Autodesk Inventor part; units mm, degrees
ref_plane "YZ Plane" through (0, 0, 0) normal (1, 0, 0) x (0, 1, 0)
ref_plane "XZ Plane" through (0, 0, 0) normal (0, 1, 0) x (-1, 0, 0)
ref_plane "XY Plane" through (0, 0, 0) normal (0, 0, 1) x (1, 0, 0)
sketch "Sketch1" plane through (0, 0, 0) normal (0, 1, 0) x (-1, 0, 0)
  line L0 (-20, 20) -> (20, 20)
  line L1 (20, 20) -> (20, -20)
  line L2 (20, -20) -> (-20, -20)
  line L3 (-20, -20) -> (-20, 20)
  line L4 (-20, 20) -> (20, -20) construction
  line L5 (20, 20) -> (-20, -20) construction
  line L6 (18, 18) -> (-18, 18)
  line L7 (-18, 18) -> (-18, -18)
  line L8 (-18, -18) -> (18, -18)
  line L9 (18, -18) -> (18, 18)
  point P0 (0, 0)
  dimension "d19" = 40
  dimension "d20" = 40
  dimension "d21" = 2
extrude "Extrusion1" add sketch "Sketch1" along normal blind 460
equation "\"BendRadius\" = Thickness"
equation "\"BendReliefWidth\" = Thickness"
equation "\"BendReliefDepth\" = 0.5 * Thickness"
equation "\"TransitionRadius\" = BendRadius"
equation "\"JacobiRadiusSize\" = BendRadius"
equation "\"GapSize\" = Thickness"
properties part number "ДМФ 033 держатель лотка v2.0"
Geometry check sheet. Reference: the model listing, model coordinates, mm. A direction names the side the tool comes from. Coordinates: 2 decimals unless noted, no trailing zeros. Order: outer loops, then holes, each group sorted by start corner. A loop starts at its lowest first (then second) coordinate and runs counter-clockwise, first axis right, second up. Notation, with made-up numbers: (21.5, 23) - (51.5, 23) arc R35 ccw to (51.5, 56) - close; hole circle Ø4 at (-5, 55). An arc over 180 degrees is marked (long way). Use one line per item in the form item = value.
1. Scan line: line 1 (Z direction, x = -4, y = 357). Record every from-to range of solid material in increasing order.
Here are the results:
line_1 = -20 to -18, 18 to 20
2. Draft check along X on faces 1 (the face through (20, 227, 0)), 2 (the face through (-18, 227, 0)), 3 (the face through (0, 227, 20)). Enter one of: pulls with the +X half, pulls with the -X half, needs draft (parallel to the pull), parting line crosses it, or undercut.
Here are the results:
face_1 = pulls with the +X half
face_2 = undercut
face_3 = needs draft
3. Access from +Z, -Z, +X, -X, +Y, -Y to the whole of each face (thin tool, end or side, straight path). Record for faces 4 (the face through (0, 227, -18)), 5 (the face through (2, 460, -19)).
Here are the results:
face_4 = +Y, -Y
face_5 = +Z, -Z, +X, -X, +Y
4. Section check C-C (z = -7). Record the boundary of the cut face in (x, y).
Here are the results:
outline = (-20, 0) - (-18, 0) - (-18, 460) - (-20, 460) - close; (18, 0) - (20, 0) - (20, 460) - (18, 460) - close
5. Section check A-A (x = -2.5). Record the boundary of the cut face in (y, z).
Here are the results:
outline = (0, -20) - (460, -20) - (460, -18) - (0, -18) - close; (0, 18) - (460, 18) - (460, 20) - (0, 20) - close
6. Section check B-B (y = 305.5). Record the boundary of the cut face in (x, z), then the cut area to 3 significant figures.
Here are the results:
outline = (-20, -20) - (20, -20) - (20, 20) - (-20, 20) - close; hole (-18, -18) - (18, -18) - (18, 18) - (-18, 18) - close
area = 304 mm²
